Design review of the part built by this model. Coordinates are the model's own, in mm. A direction names the side the tool comes from. Give positions to 0.01 mm unless a question says otherwise; leave off trailing zeros. Loops run counter-clockwise (first coordinate to the right, second up) from the corner with the lowest first, then second, coordinate; pieces in that order, holes last. Notation, with made-up numbers: (68, 70) - (121, 70) arc R20 ccw to (121, 84) - close; hole circle Ø11 at (11.25, 7). An arc over 180 degrees is marked (long way). Write each question's results on one line, items separated by ' | '.
from build123d import *

# Parameters (mm, degrees)
IZIM1_R                = 8
KAFA_YUKSEKLIGI_DEPTH  = 10
PAH1_SIZE              = 0.5
ALTIGEN_BOSALTMA_DEPTH = 5
IZIM5_W                = 5
IZIM5_H                = 20
RADYUS1_R              = 0.25
PAH2_SIZE              = 0.25


with BuildPart() as part:
    # Çizim1 → KAFA_YUKSEKLIGI (new body)
    with BuildSketch(Plane.XY):
        Circle(IZIM1_R)
    extrude(amount=KAFA_YUKSEKLIGI_DEPTH)

    # Pah1
    pah1_edges = [part.edges().sort_by_distance(p)[0] for p in [
        (-8, 0, 10),
    ]]
    chamfer(pah1_edges, length=PAH1_SIZE)

    # Çizim2 → ALTIGEN_BOSALTMA (cut)
    with BuildSketch(Plane.XY.offset(10)):
        Polygon((-4.685, 0), (-2.3425, -4.057329017), (2.3425, -4.057329017), (4.685, 0), (2.3425, 4.057329017), (-2.3425, 4.057329017), align=None)
    extrude(amount=-ALTIGEN_BOSALTMA_DEPTH, mode=Mode.SUBTRACT)

    # Kes-Ekstrüzyon2 cone 1 section (through the dimple's axis) → Kes-Ekstrüzyon2 (revolve, cut)
    with BuildSketch(Plane(origin=(0, 0, 5), x_dir=(0, -1, 0), z_dir=(1, 0, 0))):
        Polygon((0, 0), (4.057329017, 0), (0, 0.715416575), align=None)
    revolve(axis=Axis((0, 0, 5), (0, 0, -1)), mode=Mode.SUBTRACT)

    # Çizim5 → Döndür1 (revolve)
    with BuildSketch(Plane(origin=(0, 0, 0), x_dir=(1, 0, 0), z_dir=(0, 1, 0))):
        with Locations((2.5, 10)):
            Rectangle(IZIM5_W, IZIM5_H)
    revolve(axis=Axis((0, 0, 0), (0, 0, -1)))

    # Radyus1
    radyus1_edges = [part.edges().sort_by_distance(p)[0] for p in [
        (-5, 0, 0),
    ]]
    fillet(radyus1_edges, radius=RADYUS1_R)

    # Pah2
    pah2_edges = [part.edges().sort_by_distance(p)[0] for p in [
        (-5, 0, -20),
    ]]
    chamfer(pah2_edges, length=PAH2_SIZE)


solid = part.part
(1) Insertion check: P1, Ø1.5, axis at x = 1.5, y = 1.5, coming from the +Z side; P2, Ø0.6, axis at x = 2, y = -3, coming from the +Z side; P3, Ø4, axis at y = -1, z = -4, coming from the -X side. Each pin has a flat end and moves straight along its axis. Give the tip position at first contact, or say it passes through.
Answers below:
P1: z = 4.79 | P2: z = 4.97 | P3: x = -5
(2) Draft analysis for pull direction X (two halves, no side actions). For faces 3 (the flat face through (3.2, -3.2, 10)), 4 (the cylindrical face through (-1.08, 4.88, -10.14)), 5 (the flat face through (2.14, -3.64, 5)), 6 (the flat face through (3.497, -2.057, 7.535)), state which applies: pulls with the +X half, pulls with the -X half, needs draft (parallel to the pull), parting line crosses it, or undercut.
Answers below:
face 3: needs draft | face 4: parting line crosses it | face 5: undercut | face 6: undercut
(3) Wall thickness on line 1 along Y through (x, z) = (0, -18); line 2 along Z through (x, y) = (5.5, -4.5); line 3 along Y through (x, z) = (-1.75, -12.25): over which ranges is each line inside the solid? List them lowest first. Write a range as from..to.
Answers below:
line 1: -5..5 | line 2: 0..10 | line 3: -4.68..4.68
(4) Tool access review of faces 1 (the flat face through (-2.2, -3.6, 5)), 2 (the flat face through (0, 0, -20)): name each direction out of +Z, -Z, +X, -X, +Y, -Y from which nothing blocks a thin tool from reaching the whole face with its end or side.
Answers below:
face 1: +Z | face 2: -Z, +X, -X, +Y, -Y
(5) Take a section at A-A on z = 0.5. Give the boundary of the cut face in (x, y).
Answers below:
outline: circle Ø16 at (0, 0)
